from build123d import *

# Parameters (mm, degrees)
F0_R          = 30.1625
F0_R_2        = 25.4
F1_DEPTH      = 304.8
F1_DEPTH_BACK = 6.125


# Not quite as in the source:
# - a pattern or mirror of a feature is missing from the dataset's text; its kind, count and spacing are read off the source's solid


with BuildPart() as f1:
    # F0 (on Top) → F1 (new body, two sides)
    with BuildSketch(Plane.XY) as f1_sk:
        Circle(F0_R)
        Circle(F0_R_2, mode=Mode.SUBTRACT)
    extrude(amount=F1_DEPTH)
    extrude(f1_sk.sketch, amount=-F1_DEPTH_BACK)

    # F1_copies: F1 across plane


with BuildPart() as f1_1:
    add(f1.part)
    add(f1.part.mirror(Plane(origin=(0, 0, 74.6125), x_dir=(-1, 0, 0), z_dir=(0, 0, -1))))


solid = f1_1.part
For this review, take the finished solid that the model builds, in its own axes (mm). Give positions to 0.01 mm unless a question says otherwise; leave off trailing zeros. Loops run counter-clockwise (first coordinate to the right, second up) from the corner with the lowest first, then second, coordinate; pieces in that order, holes last. Notation, with made-up numbers: (66.5, 27) -> (97.5, 27) arc R12 ccw to (97.5, 44) -> close; hole circle Ø4 at (26.25, 41.5). An arc over 180 degrees is marked (long way). One line per question, with ' | ' between items.
1) To check wall thickness, follow probe 1 along Y at (x, z) = (0, 231); probe 2 along X at (y, z) = (1, 96); probe 3 along Y at (x, z) = (2.5, 48.5). State the ranges of each line that lie inside material, in increasing order.
Resolved:
probe 1: y = -30.16 to -25.4, 25.4 to 30.16 | probe 2: x = -30.15 to -25.38, 25.38 to 30.15 | probe 3: y = -30.06 to -25.28, 25.28 to 30.06
2) Insertion check: pin 1 Ø2 at (y, z) = (-13, -5) entering from +X; pin 2 Ø10 at (x, z) = (-4.5, 231) entering from -Y; pin 3 Ø6 at (x, z) = (-19, 131) entering from -Y. Each pin has a flat end and moves straight along its axis. Give the tip position at first contact, or say it passes through.
Resolved:
pin 1: stops at x = 27.67 | pin 2: stops at y = -30.16 | pin 3: stops at y = -25.57
3) We need section A-A (x = 0). Write out the cut boundary in (y, z) (1 decimal).
Resolved:
outline: (-30.2, -155.6) -> (-25.4, -155.6) -> (-25.4, 304.8) -> (-30.2, 304.8) -> close; (25.4, -155.6) -> (30.2, -155.6) -> (30.2, 304.8) -> (25.4, 304.8) -> close
4) We need section C-C (z = 243). Write out the cut boundary in (x, y) (1 decimal).
Resolved:
outline: circle Ø60.3 at (0, 0); hole circle Ø50.8 at (0, 0)
